```python
from build123d import *

# Parameters (mm, degrees)
ESQUISSE1_W             = 26
ESQUISSE1_H             = 31
ESQUISSE1_R             = 9.5
ESQUISSE1_R_2           = 1.5
BOSS_EXTRU_1_DEPTH      = 2
ESQUISSE2_R             = 11.8
ESQUISSE2_R_2           = 9.5
BOSS_EXTRU_2_DEPTH      = 2.7
CHANFREIN1_SIZE         = 1
ESQUISSE3_R             = 12
ESQUISSE3_R_2           = 8.25
BOSS_EXTRU_3_DEPTH      = 14.3
ESQUISSE4_R             = 12
BOSS_EXTRU_4_DEPTH      = 2
ESQUISSE5_R             = 1
BOSS_EXTRU_5_DEPTH      = 15
BOSS_EXTRU_5_DEPTH_BACK = 8
CONG_1_R                = 1


with BuildPart() as part:
    # Esquisse1 → Boss.-Extru.1 (new body)
    with BuildSketch(Plane.XY):
        with Locations((3.183515483, -7.666666667)):
            Rectangle(ESQUISSE1_W, ESQUISSE1_H)
        with Locations((3.183515483, -7.666666667)):
            Circle(ESQUISSE1_R, mode=Mode.SUBTRACT)
        with Locations((-6.316484517, 4.333333333)):
            Circle(ESQUISSE1_R_2, mode=Mode.SUBTRACT)
        with Locations((12.683515483, -19.666666667)):
            Circle(ESQUISSE1_R_2, mode=Mode.SUBTRACT)
    extrude(amount=BOSS_EXTRU_1_DEPTH)

    # Esquisse2 → Boss.-Extru.2 (add)
    with BuildSketch(Plane.XY.offset(2)):
        with Locations((3.183515483, -7.666666667)):
            Circle(ESQUISSE2_R)
        with Locations((3.183515483, -7.666666667)):
            Circle(ESQUISSE2_R_2, mode=Mode.SUBTRACT)
    extrude(amount=BOSS_EXTRU_2_DEPTH)

    # Chanfrein1
    chanfrein1_edges = [part.edges().sort_by_distance(p)[0] for p in [
        (-7.816484517, 4.333333333, 2),
        (11.183515483, -19.666666667, 2),
    ]]
    chamfer(chanfrein1_edges, length=CHANFREIN1_SIZE)

    # Esquisse3 → Boss.-Extru.3 (add)
    with BuildSketch(Plane(origin=(0, 0, 0), x_dir=(-1, 0, 0), z_dir=(0, 0, -1))):
        with Locations((-3.183515483, -7.666666667)):
            Circle(ESQUISSE3_R)
        with Locations((-3.183515483, -7.666666667)):
            Circle(ESQUISSE3_R_2, mode=Mode.SUBTRACT)
    extrude(amount=BOSS_EXTRU_3_DEPTH)

    # Esquisse4 → Boss.-Extru.4 (add)
    with BuildSketch(Plane(origin=(0, 0, -14.3), x_dir=(-1, 0, 0), z_dir=(0, 0, -1))):
        with Locations((-3.183515483, -7.666666667)):
            Circle(ESQUISSE4_R)
    extrude(amount=BOSS_EXTRU_4_DEPTH)

    # Esquisse5 → Boss.-Extru.5 (add, two sides)
    with BuildSketch(Plane.XY.offset(-14.3)) as boss_extru_5_sk:
        with Locations((7.243515483, -7.666666667)):
            Circle(ESQUISSE5_R)
        with Locations((-0.876484517, -7.666666667)):
            Circle(ESQUISSE5_R)
        with Locations((3.183515483, -11.646666667)):
            Circle(ESQUISSE5_R)
    extrude(amount=BOSS_EXTRU_5_DEPTH)
    extrude(boss_extru_5_sk.sketch, amount=-BOSS_EXTRU_5_DEPTH_BACK)

    # Congé1
    cong_1_edges = [part.edges().sort_by_distance(p)[0] for p in [
        (6.243515483, -7.666666667, 0.7),
        (-1.876484517, -7.666666667, 0.7),
        (2.183515483, -11.646666667, 0.7),
    ]]
    fillet(cong_1_edges, radius=CONG_1_R)


solid = part.part
```
Could you check a few things on this model? Use its own coordinates, in mm. A direction names the side the tool comes from. Coordinates: 2 decimals unless noted, no trailing zeros. Loops run counter-clockwise (first coordinate to the right, second up) from the corner with the lowest first, then second, coordinate; pieces in that order, holes last. Notation, with made-up numbers: M -27.75,31 L 11.25,31 A21 cw 11.25,69 Z; hole C -22.5,-2 d1. An arc over 180 degrees is marked long. Put each result on its own line as item: value. Start each with the question number.
(1) Thinking about a two-plate mould opening in X: for faces 4 (the face through (8.628, -18.135, 3.331)), 5 (the face through (14.114, -19.216, 0.493)), 6 (the face through (3, -12, -22.3)), which applies, pulls with the +X half, pulls with the -X half, needs draft (parallel to the pull), parting line crosses it, or undercut?
(2) Suppose I cut it at A-A on z = -6.75. Please give me the cut outline in (x, y), then the cut area to 3 significant figures.
(3) For faces 1 (the face through (9.264, -2.091, -7.05)), 2 (the face through (-0.415, -8.554, -19.258)), 3 (the face through (16.184, -8, 1)), which set-ups out of +Z, -Z, +X, -X, +Y, -Y let a thin tool reach every point of the face, with its end or its side?
(4) Suppose I cut it at C-C on z = -19.5. Please give me the cut outline in (x, y), then the cut area to 3 significant figures.
(5) I need wall thicknesses on line 1 (Y direction, x = 4, z = -9.5); line 2 (Y direction, x = 7.75, z = -2.25); line 3 (Z direction, x = -8.5, y = -19). Which ranges of each line are inside material? Lowest first, please. Write a range as from..to.
(6) Will these pins go through, and if not, where does the flat tip stop? P1, Ø1.5, axis at y = -16, z = -2.5, coming from the -X side; P2, Ø13, axis at x = 3, y = -6.5, coming from the +Z side; P3, Ø1, axis at y = -15, z = -4, coming from the +X side; P4, Ø2.5, axis at x = 12.68, y = -19.67, coming from the +Z side.
(7) Suppose I cut it at B-B on y = -15. Please give me the cut outline in (x, z), then the cut area to 3 significant figures.
Solutions:
1. face 4: parting line crosses it
1. face 5: undercut
1. face 6: needs draft
2. outline: C 3.18,-7.67 d24; C -0.88,-7.67 d2; C 3.18,-11.65 d2; C 7.24,-7.67 d2; hole C 3.18,-7.67 d16.5
2. area: 248 mm2
3. face 1: +Z
3. face 2: -Z
3. face 3: +Z, -Z, +X, +Y, -Y
4. outline: C -0.88,-7.67 d2; C 3.18,-11.65 d2; C 7.24,-7.67 d2
4. area: 9.42 mm2
5. line 1: y = -19.64..-15.88, -12.22..-11.07, 0.54..4.31
5. line 2: y = -18.76..-14.54, -8.53..-6.8, -0.8..3.43
5. line 3: z = 0..2
6. P1: stops at x = -6.12
6. P2: stops at z = 0.7
6. P3: stops at x = 13.05
6. P4: passes through
7. outline: M -9.82,0 L -6.32,0 L -6.32,-16.3 L 12.68,-16.3 L 12.68,0 L 16.18,0 L 16.18,2 L 12.43,2 L 12.43,4.7 L 9.22,4.7 L 9.22,0 L 6.96,0 L 6.96,-14.3 L -0.6,-14.3 L -0.6,0 L -2.86,0 L -2.86,4.7 L -6.06,4.7 L -6.06,2 L -9.82,2 Z
7. area: 247 mm2
